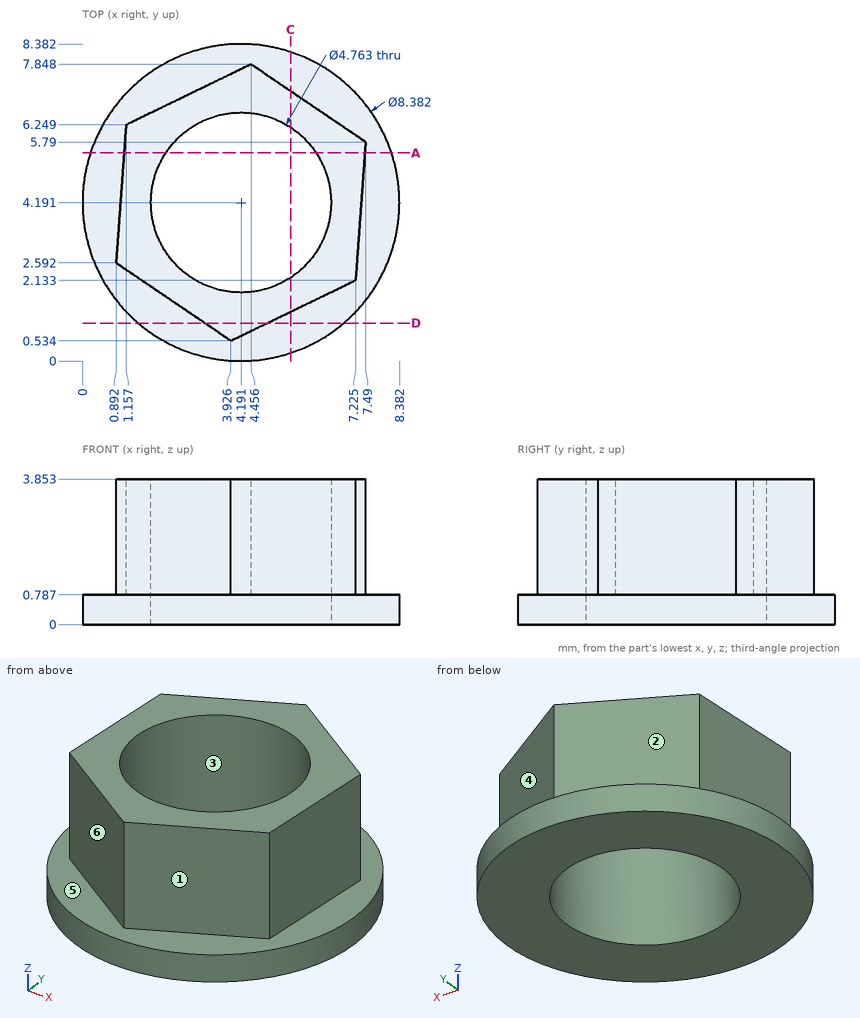
Print and shaded views of the part. All mm, measured from the part's lowest x, y and z. A direction names the side the tool comes from. Give positions to 0.01 mm unless a question says otherwise; leave off trailing zeros. Order: outer loops, then holes, each group sorted by start corner. A loop starts at its lowest first (then second) coordinate and runs counter-clockwise, first axis right, second up. Notation, with made-up numbers: M -33.75,30 L -16.75,30 A38 ccw -16.75,68 Z; hole C -1.5,20.5 d3. An arc over 180 degrees is marked long. Use one line per item in the form item = value.
Q1. Which spindle directions (+Z, -Z, +X, -X, +Y, -Y) get a long thin tool onto all of the face, cutting with end or side? Do the marked faces 4, 5 and 6. Say none if no direction does.
Conclusion:
face_4 = +Z, +X, +Y
face_5 = +Z
face_6 = +Z, -X, -Y
Q2. Slice it at C-C, the plane x = 5.5. Write the cut outline in (y, z).
Conclusion:
outline = M 0.21,0 L 2.2,0 L 2.2,3.85 L 1.3,3.85 L 1.3,0.79 L 0.21,0.79 Z; M 6.18,0 L 8.17,0 L 8.17,0.79 L 7.14,0.79 L 7.14,3.85 L 6.18,3.85 Z
Q3. Pull direction Y, two halves, no side cores. Call the marked faces 1, 2 and 3: released by +Y, released by -Y, zero draft, split by the parting line, or undercut.
Conclusion:
face_1 = released by -Y
face_2 = released by +Y
face_3 = undercut
Q4. Slice it at D-D, the plane y = 1. Write the cut outline in (x, z) (1 decimal).
Conclusion:
outline = M 1.5,0 L 6.9,0 L 6.9,0.8 L 4.9,0.8 L 4.9,3.9 L 3.2,3.9 L 3.2,0.8 L 1.5,0.8 Z
Q5. Wall check: probe 1 along X at (y, z) = (2.25, 0.2) (1 decimal); probe 2 along Z at (x, y) = (7.5, 6.25); probe 3 along Y at (x, z) = (3, 1.95) (1 decimal). Give the ranges that are in metal, low to high.
Conclusion:
probe_1 = 0.5 to 2.8, 5.6 to 7.9
probe_2 = 0 to 0.79
probe_3 = 1.2 to 2.1, 6.3 to 7.1
Q6. Slice it at A-A, the plane y = 5.5. Write the cut outline in (x, z).
Conclusion:
outline = M 0.21,0 L 2.2,0 L 2.2,3.85 L 1.1,3.85 L 1.1,0.79 L 0.21,0.79 Z; M 6.18,0 L 8.17,0 L 8.17,0.79 L 7.47,0.79 L 7.47,3.85 L 6.18,3.85 Z
Q7. Pin check, flat tips, straight feed: P1, Ø1.5, axis at y = 7, z = 2.5, coming from the +X side; P2, Ø1, axis at x = 1.5, z = 1, coming from the +Y side (1 decimal); P3, Ø2.5, axis at x = 4.5, y = 4.5, coming from the +Z side. Stop position of each tip, or through.
Conclusion:
P1 = 6.81
P2 = 7.7
P3 = through
